Design review of the part built by this model. Coordinates are the model's own, in mm. A direction names the side the tool comes from. Give positions to 0.01 mm unless a question says otherwise; leave off trailing zeros. Write each loop counter-clockwise with the first axis right and the second up, starting at its lowest first coordinate (ties: lowest second). Pieces come first, ordered by that corner, then holes. Notation, with made-up numbers: M -9,-2 L 9,-2 A23 cw 9,29 Z; hole C 81.5,64.25 d2. An arc over 180 degrees is marked long. One line per item, written item: value. Start each with the question number.
```python
from build123d import *

# Parameters (mm, degrees)
ESBO_O1_W                = 17
ESBO_O1_H                = 35
RESSALTO_EXTRUS_O1_DEPTH = 1.5
CORTE_EXTRUS_O1_REACH    = 21.685
ESBO_O2_W                = 13
ESBO_O2_H                = 23
CORTE_EXTRUS_O2_REACH    = 21.685
ESBO_O3_R                = 0.85
FILETE1_R                = 2
ESBO_O5_W                = 13
ESBO_O5_H                = 35
RESSALTO_EXTRUS_O2_DEPTH = 2
CORTE_EXTRUS_O3_REACH    = 27.758
ESBO_O6_R                = 1.75


with BuildPart() as part:
    # Esboço1 → Ressalto-extrusão1 (new, symmetric)
    with BuildSketch(Plane(origin=(0, 0, 0), x_dir=(0, 0, -1), z_dir=(1, 0, 0))):
        Rectangle(ESBO_O1_W, ESBO_O1_H)
    extrude(amount=RESSALTO_EXTRUS_O1_DEPTH, both=True)

    # Esboço2 → Corte-extrusão1 (cut, up to next)
    with BuildSketch(Plane(origin=(1.5, 0, 0), x_dir=(0, 0, -1), z_dir=(1, 0, 0)), mode=Mode.PRIVATE) as corte_extrus_o1_sk1:
        Rectangle(ESBO_O2_W, ESBO_O2_H)
    corte_extrus_o1_tool1 = extrude(corte_extrus_o1_sk1.sketch, amount=-CORTE_EXTRUS_O1_REACH, mode=Mode.PRIVATE) & part.part
    add(corte_extrus_o1_tool1.solids().sort_by_distance((1.5, 0, 0))[0], mode=Mode.SUBTRACT)

    # Esboço3 → Corte-extrusão2 (cut, up to next)
    with BuildSketch(Plane.ZY.offset(1.5), mode=Mode.PRIVATE) as corte_extrus_o2_sk1:
        with Locations((0, 14)):
            Circle(ESBO_O3_R)
    corte_extrus_o2_tool1 = extrude(corte_extrus_o2_sk1.sketch, amount=-CORTE_EXTRUS_O2_REACH, mode=Mode.PRIVATE) & part.part
    # Esboço3 → Corte-extrusão2 (cut, up to next)
    with BuildSketch(Plane.ZY.offset(1.5), mode=Mode.PRIVATE) as corte_extrus_o2_sk2:
        with Locations((0, -14)):
            Circle(ESBO_O3_R)
    corte_extrus_o2_tool2 = extrude(corte_extrus_o2_sk2.sketch, amount=-CORTE_EXTRUS_O2_REACH, mode=Mode.PRIVATE) & part.part
    add(corte_extrus_o2_tool1.solids().sort_by_distance((-1.5, 14, 0))[0], mode=Mode.SUBTRACT)
    add(corte_extrus_o2_tool2.solids().sort_by_distance((-1.5, -14, 0))[0], mode=Mode.SUBTRACT)

    # Filete1
    filete1_edges = [part.edges().sort_by_distance(p)[0] for p in [
        (0, -17.5, -8.5),
        (0, 17.5, -8.5),
    ]]
    fillet(filete1_edges, radius=FILETE1_R)

    # Esboço5 → Ressalto-extrusão2 (add)
    with BuildSketch(Plane.XY.offset(8.5)):
        with Locations((-5, 0)):
            Rectangle(ESBO_O5_W, ESBO_O5_H)
    extrude(amount=-RESSALTO_EXTRUS_O2_DEPTH)

    # Esboço6 → Corte-extrusão3 (cut, up to next)
    with BuildSketch(Plane.XY.offset(6.5), mode=Mode.PRIVATE) as corte_extrus_o3_sk1:
        with Locations(Location((-8, 14, 0), (0, 0, 180))):
            Circle(ESBO_O6_R)
    corte_extrus_o3_tool1 = extrude(corte_extrus_o3_sk1.sketch, amount=CORTE_EXTRUS_O3_REACH, mode=Mode.PRIVATE) & part.part
    # Esboço6 → Corte-extrusão3 (cut, up to next)
    with BuildSketch(Plane.XY.offset(6.5), mode=Mode.PRIVATE) as corte_extrus_o3_sk2:
        with Locations(Location((-8, -14, 0), (0, 0, 180))):
            Circle(ESBO_O6_R)
    corte_extrus_o3_tool2 = extrude(corte_extrus_o3_sk2.sketch, amount=CORTE_EXTRUS_O3_REACH, mode=Mode.PRIVATE) & part.part
    add(corte_extrus_o3_tool1.solids().sort_by_distance((-8, 14, 6.5))[0], mode=Mode.SUBTRACT)
    add(corte_extrus_o3_tool2.solids().sort_by_distance((-8, -14, 6.5))[0], mode=Mode.SUBTRACT)


solid = part.part
```
Q1. For P1, Ø2, axis at x = -8, y = -14, coming from the +Z side, flat-tipped, find the tip position at first contact; note if it passes through.
Q2. Wall thickness on line 1 (Y direction, x = -8, z = 7.2); line 2 (Y direction, x = -0.55, z = 0); line 3 (Y direction, x = 0, z = 5.75): over which ranges is each line inside the solid? List them lowest first. Write a range as from..to.
Q3. Machinability: for faces 1 (the face through (-5, 0, 8.5)), 2 (the face through (0, 0, -6.5)), which of the approach directions +Z, -Z, +X, -X, +Y, -Y give a long, thin tool a straight path to every point of the face, cutting with its end or side? Answer none if there is none.
Q4. Take a section at B-B, the plane y = -11. Give the boundary of the cut face in (x, z), then the cut area to 3 significant figures.
Q5. Take a section at C-C, the plane x = -8. Give the boundary of the cut face in (y, z), then the cut area to 3 significant figures.
Q6. Take a section at A-A, the plane z = 0. Give the boundary of the cut face in (x, y).
Q7. The part is to be moulded in two halves that separate along Y. For faces 3 (the face through (-1.5, 4, -8)), 4 (the face through (-5, 0, 6.5)), 5 (the face through (-0.02, 16.93, -7.9)), say which applies: pulls with the +Y half, pulls with the -Y half, needs draft (parallel to the pull), parting line crosses it, or undercut.
Q8. Take a section at D-D, the plane y = 14. Give the boundary of the cut face in (x, z).
Results list:
1. P1: passes through
2. line 1: y = -17.5..-15.75, -12.25..12.25, 15.75..17.5
2. line 2: y = -17.5..-14.85, -13.15..-11.5, 11.5..13.15, 14.85..17.5
2. line 3: y = -17.5..-11.5, 11.5..17.5
3. face 1: +Z, +X, -X, +Y, -Y
3. face 2: +X, -X
4. outline: M -11.5,6.5 L 1.5,6.5 L 1.5,8.5 L -11.5,8.5 Z; M -1.5,-8.5 L 1.5,-8.5 L 1.5,-6.5 L -1.5,-6.5 Z
4. area: 32.0 mm^2
5. outline: M -17.5,6.5 L -15.75,6.5 L -15.75,8.5 L -17.5,8.5 Z; M -12.25,6.5 L 12.25,6.5 L 12.25,8.5 L -12.25,8.5 Z; M 15.75,6.5 L 17.5,6.5 L 17.5,8.5 L 15.75,8.5 Z
5. area: 56.0 mm^2
6. outline: M -1.5,-17.5 L 1.5,-17.5 L 1.5,-14.85 L -1.5,-14.85 Z; M -1.5,-13.15 L 1.5,-13.15 L 1.5,-11.5 L -1.5,-11.5 Z; M -1.5,11.5 L 1.5,11.5 L 1.5,13.15 L -1.5,13.15 Z; M -1.5,14.85 L 1.5,14.85 L 1.5,17.5 L -1.5,17.5 Z
7. face 3: needs draft
7. face 4: undercut
7. face 5: pulls with the +Y half
8. outline: M -11.5,6.5 L -9.75,6.5 L -9.75,8.5 L -11.5,8.5 Z; M -6.25,6.5 L -1.5,6.5 L -1.5,0.85 L 1.5,0.85 L 1.5,8.5 L -6.25,8.5 Z; M -1.5,-8.5 L 1.5,-8.5 L 1.5,-0.85 L -1.5,-0.85 Z
